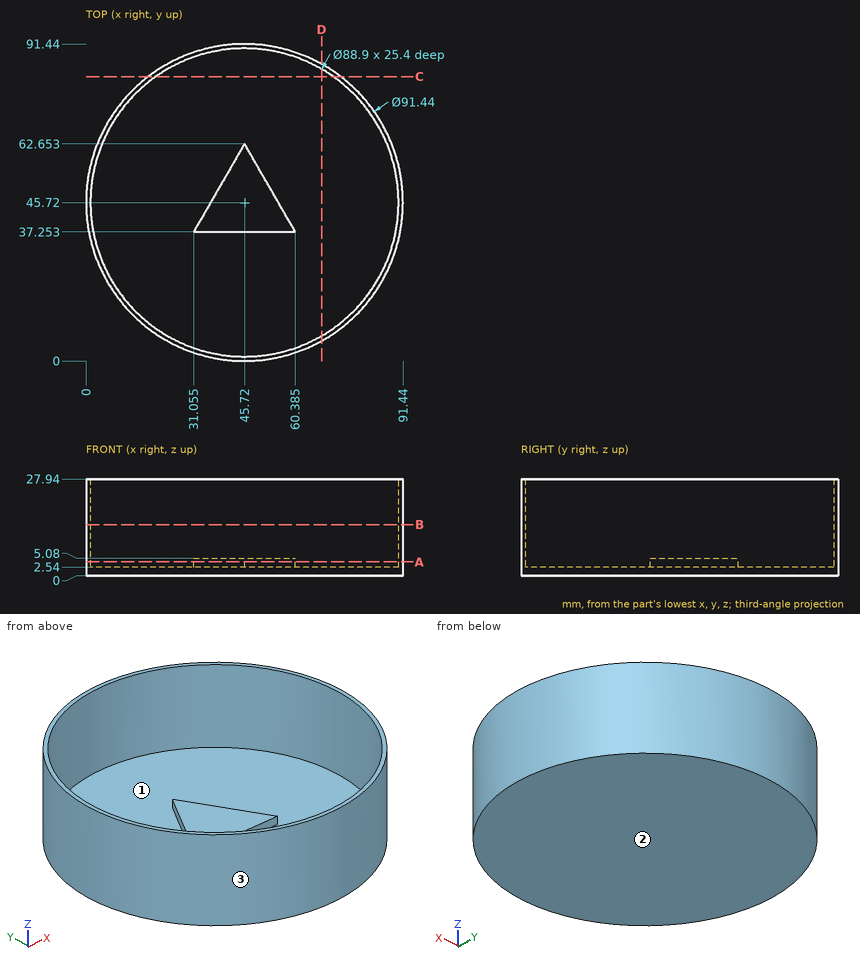
Print and shaded views of the part. All mm, measured from the part's lowest x, y and z. Coordinates: 2 decimals unless noted, no trailing zeros. Order: outer loops, then holes, each group sorted by start corner. A loop starts at its lowest first (then second) coordinate and runs counter-clockwise, first axis right, second up. Notation, with made-up numbers: M 28,-32 L 60,-32 A17 ccw 60,0 Z; hole C 28,11.25 d11. An arc over 180 degrees is marked long. Write each question's results on one line, items separated by ' | '. Start each with the question number.
Q1. Pull direction X, two halves, no side cores. Call the marked faces 1, 2 and 3: +X half, -X half, draft (parallel to the pull), parting line (faces both ways), or undercut.
Q2. Cut at B-B (z = 14.75). List the corners of the cut face in (x, y).
Q3. Flat gauge pins, fed straight in: P1, Ø3, axis at y = 31, z = 12, coming from the -X side; P2, Ø8, axis at x = 24.5, y = 61, coming from the +Z side; P3, Ø12, axis at y = 73, z = 17.5, coming from the +X side (1 decimal). Where does each tip first touch, or does it go through?
Q4. Drill centre lines: probe 1 along Y at (x, z) = (45.72, 15.25); probe 2 along Y at (x, z) = (65, 5.25) (1 decimal); probe 3 along Z at (x, y) = (60.5, 69). Where is each one in solid material? Low to high. Write a range as from..to.
Q5. Cut at A-A (z = 4). Count the separate pieces of the cut face and the enclosed holes in it.
Q6. Cut at C-C (y = 82). List the corners of the cut face in (x, z), then the cut area to 3 significant figures.
Q7. Cut at D-D (x = 68). List the corners of the cut face in (y, z), then the cut area to 3 significant figures.
Found:
1) face 1: undercut | face 2: draft | face 3: parting line
2) outline: C 45.72,45.72 d91.44; hole C 45.72,45.72 d88.9
3) P1: x = 1.95 | P2: z = 2.54 | P3: x = 86.2
4) probe 1: 0..1.27, 90.17..91.44 | probe 2: 4.3..5.7, 85.8..87.2 | probe 3: 0..2.54
5) separate pieces: 2 | enclosed holes: 1
6) outline: M 17.9,0 L 73.54,0 L 73.54,27.94 L 71.4,27.94 L 71.4,2.54 L 20.04,2.54 L 20.04,27.94 L 17.9,27.94 Z | area: 250 mm²
7) outline: M 5.8,0 L 85.64,0 L 85.64,27.94 L 84.18,27.94 L 84.18,2.54 L 7.26,2.54 L 7.26,27.94 L 5.8,27.94 Z | area: 277 mm²
